The model under review builds one solid part; all positions refer to its coordinate system, in mm. A direction names the side the tool comes from. Round coordinates to 2 decimals unless told otherwise and drop trailing zeros. Order: outer loops, then holes, each group sorted by start corner. A loop starts at its lowest first (then second) coordinate and runs counter-clockwise, first axis right, second up.
1) Machinability: for faces 5 (the face through (20, 0, 5)), 6 (the face through (0, 0, 0)), which of the approach directions +Z, -Z, +X, -X, +Y, -Y give a long, thin tool a straight path to every point of the face, cutting with its end or side? Answer none if there is none.
2) Consider section D-D (x = 21.5). Give the boundary of the cut face in (y, z), then the cut area to 3 significant figures.
3) Mouldability with a two-part tool opening along X and no side actions: class faces 1 (the face through (2.5, 0, 5)), 2 (the face through (23.846, 7.509, 4.93)), 3 (the face through (0, 0, 10)), 4 (the face through (-2.5, 0, 5)) as pulls with the +X half, pulls with the -X half, needs draft (parallel to the pull), parting line crosses it, or undercut.
4) Consider section A-A (y = 0). Give the boundary of the cut face in (x, z), then the cut area to 3 significant figures.
5) Clearance check with flat-ended pins moving along their axes: P1, Ø6, axis at y = -16, z = 5.5, coming from the +X side; P2, Ø3, axis at y = 6, z = 6, coming from the -X side; P3, Ø2, axis at y = -14.5, z = 8.5, coming from the -X side; P4, Ø5, axis at y = -2, z = 6, coming from the +X side. State where each tip first meets the part, or that it passes through.
6) To check wall thickness, follow L1, parallel to X at y = -11.5, z = 5; L2, parallel to X at y = -0.5, z = 4 (3 decimals); L3, parallel to Y at x = 13, z = 9.5. State the ranges of each line that lie inside material, in increasing order.
7) Consider section C-C (y = 16). Give the boundary of the cut face in (x, z).
8) Consider section B-B (z = 5.5). Give the boundary of the cut face in (x, y).
from build123d import *

# Parameters (mm, degrees)
F0_R     = 25
F1_DEPTH = 10
F3_DEPTH = 10


with BuildPart() as f1:
    # F0 (on Top) → F1 (new body)
    with BuildSketch(Plane.XY):
        Circle(F0_R)
    extrude(amount=F1_DEPTH)

    # F2 (on face) → F3 (cut)
    with BuildSketch(Plane.XY.offset(10)):
        with BuildLine():
            ThreePointArc((-2.499999, 19.843135), (-20, 0), (-2.499999, -19.843135))
            Line((-2.499999, -19.843135), (-2.499999, 19.843135))
        make_face()
        with BuildLine():
            ThreePointArc((2.500001, -19.843142), (20.000003, -7e-06), (2.500001, 19.843128))
            Line((2.500001, 19.843128), (2.500001, -19.843142))
        make_face()
    extrude(amount=-F3_DEPTH, mode=Mode.SUBTRACT)


solid = f1.part
Answer below:
1. face 5: +Z, -Z
1. face 6: -Z, +X, -X, +Y, -Y
2. outline: (-12.76, 0) - (12.76, 0) - (12.76, 10) - (-12.76, 10) - close
2. area: 255 mm2
3. face 1: undercut
3. face 2: parting line crosses it
3. face 3: needs draft
3. face 4: undercut
4. outline: (-25, 0) - (-20, 0) - (-20, 10) - (-25, 10) - close; (-2.5, 0) - (2.5, 0) - (2.5, 10) - (-2.5, 10) - close; (20, 0) - (25, 0) - (25, 10) - (20, 10) - close
4. area: 150 mm2
5. P1: stops at x = 21.35
5. P2: stops at x = -24.59
5. P3: stops at x = -21.04
5. P4: stops at x = 25
6. L1: x = -22.2 to -16.36, -2.5 to 2.5, 16.36 to 22.2
6. L2: x = -24.995 to -19.994, -2.5 to 2.5, 19.994 to 24.995
6. L3: y = -21.35 to -15.2, 15.2 to 21.35
7. outline: (-19.21, 0) - (-12, 0) - (-12, 10) - (-19.21, 10) - close; (-2.5, 0) - (2.5, 0) - (2.5, 10) - (-2.5, 10) - close; (12, 0) - (19.21, 0) - (19.21, 10) - (12, 10) - close
8. outline: circle Ø50 at (0, 0); hole (-2.5, -19.84) - (-2.5, 19.84) arc R20 ccw to start; hole (2.5, -19.84) arc R20 ccw to (2.5, 19.84) - close
